from build123d import *

# Parameters (mm, degrees)
SKETCH_W        = 50
SKETCH_H        = 75
PAD_DEPTH       = 18
SKETCH001_R     = 17.8
POCKET_DEPTH    = 18.001
SKETCH005_W     = 25.040878
SKETCH005_H     = 24.535461
SKETCH005_W_2   = 12.208063
SKETCH005_H_2   = 50.590956
POCKET001_DEPTH = 5
POCKET002_DEPTH = 25
SKETCH003_W     = 3
SKETCH003_H     = 5.8
POCKET003_DEPTH = 50.001
SKETCH004_W     = 72.31723
SKETCH004_H     = 2
POCKET004_DEPTH = 17.8
CHAMFER_SIZE    = 10
FILLET_R        = 7
FILLET001_R     = 1
FILLET002_R     = 2


with BuildPart() as part:
    # Sketch → Pad (new body)
    with BuildSketch(Plane.XY):
        Rectangle(SKETCH_W, SKETCH_H)
    extrude(amount=PAD_DEPTH)

    # Sketch001 → Pocket (cut, through all)
    with BuildSketch(Plane.XY.offset(18)):
        with Locations((0, -15.5)):
            Circle(SKETCH001_R)
    extrude(amount=-POCKET_DEPTH, mode=Mode.SUBTRACT)

    # Sketch005 → Pocket001 (cut)
    with BuildSketch(Plane.XZ.offset(37.5)):
        with Locations((-27.520439, 8.08709)):
            Rectangle(SKETCH005_W, SKETCH005_H)
        with Locations((21.104031, -3.872155)):
            Rectangle(SKETCH005_W_2, SKETCH005_H_2)
    extrude(amount=-POCKET001_DEPTH, mode=Mode.SUBTRACT)

    # Sketch002 → Pocket002 (cut)
    with BuildSketch(Plane.XZ.offset(32.5)):
        Polygon((-22.267329, 9), (-20.004588, 11.262742), (-17.741846, 9), (-20.004588, 6.737258), align=None)
        Polygon((17.895693, 9), (20.158435, 11.262742), (22.421177, 9), (20.158435, 6.737258), align=None)
    extrude(amount=-POCKET002_DEPTH, mode=Mode.SUBTRACT)

    # Sketch003 → Pocket003 (cut, through all)
    with BuildSketch(Plane.YZ.offset(25)):
        with Locations((-9.5, 9)):
            Rectangle(SKETCH003_W, SKETCH003_H)
    extrude(amount=-POCKET003_DEPTH, mode=Mode.SUBTRACT)

    # Sketch004 → Pocket004 (cut)
    with BuildSketch(Plane.XY.offset(18)):
        with Locations((-0.391915, -15.598591)):
            Rectangle(SKETCH004_W, SKETCH004_H)
    extrude(amount=-POCKET004_DEPTH, mode=Mode.SUBTRACT)

    # Chamfer
    chamfer_edges = [part.edges().sort_by_distance(p)[0] for p in [
        (0, 37.5, 18),
    ]]
    chamfer(chamfer_edges, length=CHAMFER_SIZE)

    # Fillet
    fillet_edges = [part.edges().sort_by_distance(p)[0] for p in [
        (0, 37.5, 8),
    ]]
    fillet(fillet_edges, radius=FILLET_R)

    # Fillet001
    fillet001_edges = [part.edges().sort_by_distance(p)[0] for p in [
        (0, 27.5, 18),
    ]]
    fillet(fillet001_edges, radius=FILLET001_R)

    # Fillet002
    fillet002_edges = [part.edges().sort_by_distance(p)[0] for p in [
        (15, -32.5, 9),
        (25, -32.5, 9),
        (15, -37.5, 9),
        (-15, -32.5, 9),
        (-15, -37.5, 9),
        (-25, -32.5, 9),
    ]]
    fillet(fillet002_edges, radius=FILLET002_R)


solid = part.part
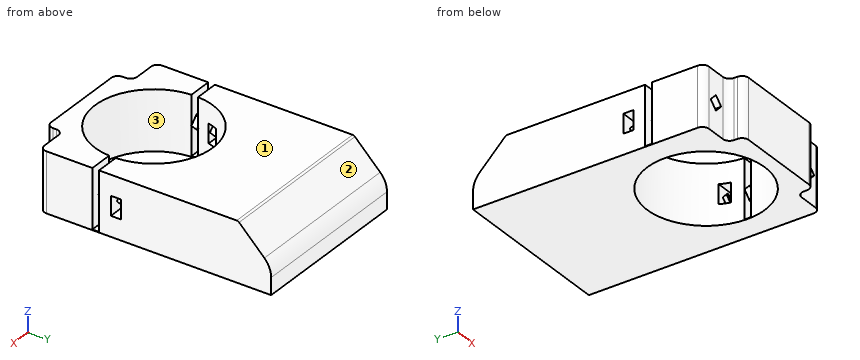
Part model, mm, in its own coordinate system. Face numbers are marked on the shaded views. Coordinates: 2 decimals unless noted, no trailing zeros. Loops run counter-clockwise (first coordinate to the right, second up) from the corner with the lowest first, then second, coordinate; pieces in that order, holes last. Notation, with made-up numbers: (-29.75, 89) - (-7.75, 89) arc R26 cw to (-7.75, 113) - close; hole circle Ø10 at (8, 49.5). An arc over 180 degrees is marked (long way). Write each question's results on one line, items separated by ' | '. Start each with the question number.
Q1. Drop flat-ended pins along their axis: pin 1 Ø6.5 at (x, z) = (21, 8) entering from -Y; pin 2 Ø5 at (x, z) = (-16, 6.5) entering from -Y; pin 3 Ø10 at (x, z) = (12.5, 10.5) entering from +Y. Give the stop position or say it passes through.
Q2. Slice it at B-B on y = -15.5. Give the cut face in (x, z), and give its area (3 significant figures).
Q3. Slice it at A-A on z = 16.5. Give the cut face in (x, y).
Q4. Slice it at C-C on x = 0. Give the cut face in (y, z).
Q5. Two-plate mould, pull along Y, no slides. Class the marked faces 1, 2 and 3: +Y half, -Y half, draft (parallel to the pull), parting line (faces both ways), or undercut.
Q6. Probe line 1 along Y through (x, z) = (-13.5, 10.25); line 2 along Y through (x, z) = (-19.5, 5.25); line 3 along X through (y, z) = (-26, 13). List the from-to ranges inside material, lowest first.
Q7. Slice it at D-D on x = -6. Give the cut face in (y, z).
Answer:
1) pin 1: stops at y = -32.5 | pin 2: stops at y = -37.44 | pin 3: stops at y = 37.49
2) outline: (-25, 0) - (-17.8, 0) - (-17.8, 0.2) - (-25, 0.2) - close; (17.8, 0) - (25, 0) - (25, 0.2) - (17.8, 0.2) - close | area: 2.88 mm2
3) outline: (-25, -30.5) arc R2 ccw to (-23, -32.5) - (-17, -32.5) arc R2 cw to (-15, -34.5) - (-15, -35.5) arc R2 ccw to (-13, -37.5) - (13, -37.5) arc R2 ccw to (15, -35.5) - (15, -34.5) arc R2 cw to (17, -32.5) - (23, -32.5) arc R2 ccw to (25, -30.5) - (25, -16.6) - (17.77, -16.6) arc R17.8 cw to (-17.77, -16.6) - (-25, -16.6) - close; (-25, -14.6) - (-17.78, -14.6) arc R17.8 cw to (17.78, -14.6) - (25, -14.6) - (25, 29) - (-25, 29) - close
4) outline: (-37.5, 0) - (-33.3, 0) - (-33.3, 18) - (-37.5, 18) - close; (2.3, 0) - (37.5, 0) - (37.5, 5.1) arc R7 ccw to (35.45, 10.05) - (27.79, 17.71) arc R1 ccw to (27.09, 18) - (2.3, 18) - close
5) face 1: draft | face 2: +Y half | face 3: undercut
6) line 1: y = -37.44 to -27.1, -3.9 to 35.25 | line 2: y = -32.5 to -16.6, -14.6 to 37.5 | line 3: x = -25 to -14.37, 14.37 to 25
7) outline: (-37.5, 0) - (-32.26, 0) - (-32.26, 18) - (-37.5, 18) - close; (1.26, 0) - (37.5, 0) - (37.5, 5.1) arc R7 ccw to (35.45, 10.05) - (27.79, 17.71) arc R1 ccw to (27.09, 18) - (1.26, 18) - close
